Read the model definition and answer for the solid it produces. Units are mm, in the model's axes. A direction names the side the tool comes from. Give positions to 0.01 mm unless a question says otherwise; leave off trailing zeros. Loops run counter-clockwise (first coordinate to the right, second up) from the corner with the lowest first, then second, coordinate; pieces in that order, holes last. Notation, with made-up numbers: (42.25, 17.25) - (77.25, 17.25) arc R31 cw to (77.25, 53.25) - close; hole circle Ø6 at (75.5, -1.75). An arc over 180 degrees is marked (long way). Use a Markdown table: item, result. Add a question column.
Item 1: Which of the six approach directions +Z, -Z, +X, -X, +Y, -Y give full straight-line access (tool end or side, diameter ignored) to faces 1 (the face through (8, 0, -66)), 2 (the face through (-4, -4.5, -89)), 3 (the face through (-163.267, -2.218, -85.659)), 4 (the face through (-121.154, 0.986, -125.253))?
Item 2: Consider probe 1 along X at (y, z) = (-0.25, -120); probe 2 along Z at (x, y) = (-11, -1); probe 3 along X at (y, z) = (-5.5, -3.5). Determine where each line is inside the solid, lowest interval first. Write a range as [from, to].
Item 3: Each of these flat-tipped pins is pushed along its axis until it touches: P1, Ø1.6, axis at x = -127, y = -1, coming from the +Z side; P2, Ø2.5, axis at x = -3.5, z = -3.5, coming from the -Y side; P3, Ø3.5, axis at x = -4, z = -86.5, coming from the -Y side. Where does it stop, or does it pass through?
Item 4: For a pull along Z with two mould halves and no side action, classify faces 5 (the face through (-25.507, 0.986, -123.33)), 6 (the face through (-94, 0, -139)), 7 (the face through (7.945, -1.014, -16.389)) as +Z half, -Z half, draft (parallel to the pull), parting line (faces both ways), or undercut.
Item 5: A cutting plane is placed at A-A (z = -123). Determine the outline of the cut face in (x, y), plus the area to 3 significant figures.
Item 6: A cutting plane is placed at B-B (z = -55.5). Give the number of separate pieces and of enclosed holes in the cut face, plus the area to 3 significant figures.
Autodesk Inventor part; units mm, degrees
ref_plane "YZ Plane" through (0, 0, 0) normal (1, 0, 0) x (0, 1, 0)
ref_plane "XZ Plane" through (0, 0, 0) normal (0, 1, 0) x (-1, 0, 0)
ref_plane "XY Plane" through (0, 0, 0) normal (0, 0, 1) x (1, 0, 0)
sketch "Skizze1" plane through (0, 0, 0) normal (0, 1, 0) x (-1, 0, 0)
  line L0 (0, 0) -> (170, 0)
  line L1 (170, 0) -> (170, -140)
  line L2 (170, -140) -> (0, -140)
  line L3 (0, -140) -> (0, 0)
  circle A0 centre (150, -123) radius 7.5
  circle A1 centre (114, -123) radius 7.5
  circle A2 centre (73.5, -123) radius 7.5
  circle A3 centre (33, -123) radius 7.5
  line L4 (153, -30) -> (136, -30)
  line L5 (136, -30) -> (136, -64)
  line L6 (136, -64) -> (153, -64)
  line L7 (153, -64) -> (153, -30)
  circle A4 centre (121.5, -55.5) radius 6.5
  line L8 (150, -123) -> (0, -123) construction
  dimension "d0" = 170
  dimension "d1" = 140
  dimension "d2" = 15
  dimension "d3" = 123
  dimension "d4" = 20
  dimension "d8" = 56
  dimension "d9" = 96.5
  dimension "d10" = 137
  dimension "d11" = 17
  dimension "d12" = 34
  dimension "d13" = 30
  dimension "d14" = 17
  dimension "d15" = 13
  dimension "d17" = 48.5
  dimension "d100" = 25.5
extrude "Extrusion1" add sketch "Skizze1" along normal blind 2
chamfer "Fase1" distance 2 angle 45 4 edges at (-153, 2, -47) (-144.5, 2, -64) (-136, 2, -47) (-144.5, 2, -30)
sketch "Skizze2" plane through (0, 0, 0) normal (0, -1, 0) x (1, 0, 0)
  circle A0 centre (-101.8979, -9.7616) radius 3.5
  circle A1 centre (-3.5, -87) radius 3.5
  circle A2 centre (-3.5, -3.5) radius 3.5
  line L0 (0, 0) -> (0, -140)
  line L1 (0, -140) -> (-170, -140)
  line L2 (-170, 0) -> (0, 0)
  circle A3 centre (-166.5, -87) radius 3.5
  line L3 (-170, -140) -> (-170, 0)
  dimension "d23" = 7
  dimension "d24" = 7
  dimension "d25" = 7
  dimension "d26" = 3.5
  dimension "d28" = 3.5
  dimension "d29" = 3.5
  dimension "d30" = 7
  dimension "d31" = 3.5
  dimension "d32" = 87
  dimension "d33" = 87
extrude "Extrusion2" add sketch "Skizze2" along normal blind 4.5 contours A0 | A1 | A3 | A2
sketch "Skizze3" plane through (-101.8979, -4.5, -9.7616) normal (0, -1, 0) x (1, 0, 0)
  circle A0 centre (0, 0) radius 3.5
  circle A1 centre (98.3979, 6.2616) radius 3.5
  point P0 (101.8979, 9.7616)
extrude "Extrusion3" add sketch "Skizze3" along normal blind 2.5
sketch "Skizze4" plane through (-166.5, -4.5, -87) normal (0, -1, 0) x (1, 0, 0)
  circle A0 centre (163, 0) radius 3.5
  point P0 (166.5, 87)
hole "Bohrung1" at (-3.5, -4.5, -87) direction (0, 1, 0) diameter 3 depth 5
sketch "Skizze5" plane through (-3.5, -7, -3.5) normal (0, -1, 0) x (1, 0, 0)
  circle A0 centre (0, 0) radius 3.5
  point P0 (3.5, 3.5)
hole "Bohrung2" at (-3.5, -7, -3.5) direction (0, 1, 0) diameter 3 depth 7
sketch "Skizze6" plane through (-101.8979, -7, -9.7616) normal (0, -1, 0) x (1, 0, 0)
  circle A0 centre (0, 0) radius 3.5
  point P0 (101.8979, 9.7616)
hole "Bohrung3" at (-101.8979, -7, -9.7616) direction (0, 1, 0) diameter 3 depth 7
sketch "Skizze7" plane through (-166.5, -4.5, -87) normal (0, -1, 0) x (1, 0, 0)
  circle A0 centre (0, 0) radius 3.5
  point P0 (166.5, 87)
hole "Bohrung4" at (-166.5, -4.5, -87) direction (0, 1, 0) diameter 3 depth 5
sketch "Skizze8" plane through (0, 0, 0) normal (0, -1, 0) x (1, 0, 0)
  line L0 (0, -140) -> (-170, -140)
  line L1 (0, -140) -> (-8, -140)
  line L2 (-8, -140) -> (-8, -20)
  line L3 (-8, -20) -> (0, -20)
  line L4 (0, -20) -> (0, -140)
  circle A0 centre (-33, -123) radius 7.5
  circle A1 centre (-150, -123) radius 7.5
  line L5 (-170, -24.5) -> (-175, -24.5)
  line L6 (-175, -24.5) -> (-175, -144.5)
  line L7 (-175, -144.5) -> (-170, -144.5)
  line L8 (-170, -144.5) -> (-170, -24.5)
  line L9 (-170, -140) -> (-170, -87)
  line L10 (-175, -24.5) -> (-1, -24.5)
  line L11 (-1, -24.5) -> (-1, -12.2606)
  line L12 (-1, -12.2606) -> (-175, -12.2606)
  line L13 (-175, -12.2606) -> (-175, -24.5)
  point P0 (0, 0)
  point P1 (0, 0)
  point P2 (-1, -20)
  dimension "d66" = 25
  dimension "d67" = 25
extrude "Extrusion4" add sketch "Skizze8" against normal blind 2 contours L0 L2 L10 L11 L3 L4 | L8 L7 L6 L5 | L10 L5 L13 L12 L11 L3 L2 | L2 L3 L11 L10
sketch "Skizze9" plane through (0, 0, 0) normal (0, -1, 0) x (1, 0, 0)
  arc A0 (0, -3.5) -> (-3.5, 0) centre (-3.5, -3.5) ccw
  circle A1 centre (-3.5, -87) radius 3.5
  circle A2 centre (-101.8979, -9.7616) radius 3.5
  circle A3 centre (-150, -123) radius 7.5
  circle A4 centre (-114, -123) radius 7.5
  circle A5 centre (-73.5, -123) radius 7.5
  circle A6 centre (-33, -123) radius 7.5
  circle A7 centre (-121.5, -55.5) radius 6.5
  line L0 (-153, -30) -> (-153, -64)
  line L1 (-136, -30) -> (-153, -30)
  line L2 (-136, -64) -> (-136, -30)
  line L3 (-153, -64) -> (-136, -64)
  circle A8 centre (-166.5, -87) radius 3.5
  line L4 (9.3, -137.3) -> (-175, -137.3)
  line L5 (9.3, -137.3) -> (9.3, -14.9606)
  line L6 (9.3, -14.9606) -> (-175, -14.9606)
  line L7 (-175, -14.9606) -> (-175, -137.3)
  line L8 (12, -120) -> (12, 12.2394)
  line L9 (-170, -12.2606) -> (-175, -12.2606)
  line L10 (-175, -12.2606) -> (-175, -144.5)
  line L11 (0, -140) -> (-175, -140)
  line L12 (-173, -16.9606) -> (7.3, -16.9606)
  line L13 (7.3, -16.9606) -> (7.3, -135.3)
  line L14 (7.3, -135.3) -> (-173, -135.3)
  line L15 (-173, -135.3) -> (-173, -16.9606)
  line L16 (-173, -135.3) -> (-173, -137.3)
  point P0 (0, 0)
  dimension "d81" = 127.7394
  dimension "d70" = 2.7
  dimension "d71" = 2.7
  dimension "d72" = 0
  dimension "d73" = 2.7
  dimension "d74" = 2
  dimension "d75" = 2
  dimension "d76" = 2
  dimension "d77" = 2
extrude "Extrusion5" add sketch "Skizze9" along normal blind 2 contours L4 L7 L6 L5
fillet "Rundung1" radius 4.75 2 edges at (9.3, -1, -137.3) (9.3, -1, -14.9606)
sketch "Skizze10" plane through (9.3, 0, -19.7106) normal (1, 0, 0) x (0, 0, -1)
  line L0 (117.5894, 0) -> (-4.75, 0)
  line L1 (53.6697, 0) -> (63.6697, 0)
  line L2 (63.6697, 0) -> (63.6697, -3.5)
  line L3 (63.6697, -3.5) -> (53.6697, -3.5)
  line L4 (53.6697, -3.5) -> (53.6697, 0)
  line L5 (58.6697, -3.5) -> (58.6697, 0)
  line L6 (-2.7, 2) -> (120.0394, 2)
  line L7 (0, 0) -> (117.3394, 0)
  line L8 (53.6697, -2.5) -> (63.6697, -2.5)
  point P0 (-19.7106, 0)
  dimension "d83" = 1
  dimension "d91" = 10
  dimension "d92" = 2.5
extrude "Extrusion6" add sketch "Skizze10" against normal blind 2
extrude "Extrusion7" add sketch "Skizze10" along normal blind 0.4 contours L2 L3 L5 L8 | L5 L3 L4 L8
chamfer "Fase2" distance 0.25 angle 45 2 edges at (9.7, -2.5, -78.3803) (9.7, -3.5, -78.3803)
chamfer "Fase3" distance 2 angle 30 1 edges at (-175, 2, -78.3803) measured on face at (-175, 1.3333, -57.2404)
sketch "Skizze11" plane through (9.3, 0, -19.7106) normal (1, 0, 0) x (0, 0, -1)
  line L0 (112.8394, 0) -> (112.8394, -2)
  line L1 (117.3394, 0) -> (105.2695, 0)
  line L2 (105.2695, 0) -> (105.2695, -2)
  line L3 (105.2695, -2) -> (117.3394, -2)
  line L4 (117.3394, -2) -> (117.3394, 0)
  point P0 (-19.7106, 0)
extrude "Extrusion8" cut sketch "Skizze11" against normal blind 3.2
sketch "Skizze12" plane through (4.55, -2, -137.3) normal (0, 0, -1) x (-1, 0, 0)
  line L0 (177.55, 0) -> (-2.75, 0)
  line L1 (4.55, 2) -> (179.55, 2)
  line L2 (99.55, 0) -> (84.55, 0)
  line L3 (84.55, 0) -> (84.55, 2)
  line L4 (84.55, 2) -> (99.55, 2)
  line L5 (99.55, 2) -> (99.55, 0)
  line L6 (179.55, 2) -> (179.55, 0)
  point P0 (0, 2)
  dimension "d98" = 15
  dimension "d99" = 80
properties part number "Fascia"
Geometry says:
| question | item | result |
|---|---|---|
| 1 | face 1 | +Z, -Z, +X, +Y |
| 1 | face 2 | -Z, +X, -X, -Y |
| 1 | face 3 | -Y |
| 1 | face 4 | +Y, -Y |
| 2 | probe 1 | [-175, -173], [7.3, 9.3] |
| 2 | probe 2 | [-137.3, -135.3], [-16.96, -14.96] |
| 2 | probe 3 | [-7, -5], [-2, 0] |
| 3 | P1 | z = -14.96 |
| 3 | P2 | y = 0 |
| 3 | P3 | y = -4.5 |
| 4 | face 5 | undercut |
| 4 | face 6 | draft |
| 4 | face 7 | +Z half |
| 5 | outline | (-175, -2) - (-173, -2) - (-173, 0) - (-157.5, 0) - (-157.5, 2) - (-173.85, 2) - (-175, 0) - close; (-142.5, 0) - (-121.5, 0) - (-121.5, 2) - (-142.5, 2) - close; (-106.5, 0) - (-81, 0) - (-81, 2) - (-106.5, 2) - close; (-66, 0) - (-40.5, 0) - (-40.5, 2) - (-66, 2) - close; (-25.5, 0) - (0, 0) - (0, 2) - (-25.5, 2) - close; (7.3, -2) - (9.3, -2) - (9.3, 0) - (7.3, 0) - close |
| 5 | area | 237 mm² |
| 6 | separate pieces | 4 |
| 6 | enclosed holes | 0 |
| 6 | area | 293 mm² |
